```python
from build123d import *

# Parameters (mm, degrees)
SKETCH1_W           = 400
SKETCH1_H           = 1000
SKETCH1_W_2         = 360
SKETCH1_H_2         = 960
SKETCH1_H_3         = 20
BOSS_EXTRUDE1_DEPTH = 400
SKETCH2_W           = 400
SKETCH2_H           = 1000
BOSS_EXTRUDE2_DEPTH = 10


with BuildPart() as part:
    # Sketch1 → Boss-Extrude1 (new body)
    # profile 1 of 4: a face of its own
    with BuildSketch(Plane.XY):
        with Locations((0, 500)):
            Rectangle(SKETCH1_W, SKETCH1_H)
        with Locations((0, 500)):
            Rectangle(SKETCH1_W_2, SKETCH1_H_2, mode=Mode.SUBTRACT)
    # profile 2 of 4: a face of its own
    with BuildSketch(Plane.XY):
        with Locations((0, 740)):
            Rectangle(SKETCH1_W_2, SKETCH1_H_3)
    # profile 3 of 4: a face of its own
    with BuildSketch(Plane.XY):
        with Locations((0, 500)):
            Rectangle(SKETCH1_W_2, SKETCH1_H_3)
    # profile 4 of 4: a face of its own
    with BuildSketch(Plane.XY):
        with Locations((0, 260)):
            Rectangle(SKETCH1_W_2, SKETCH1_H_3)
    extrude(amount=BOSS_EXTRUDE1_DEPTH)

    # Sketch2 → Boss-Extrude2 (add)
    with BuildSketch(Plane(origin=(0, 0, 0), x_dir=(-1, 0, 0), z_dir=(0, 0, -1))):
        with Locations((0, 500)):
            Rectangle(SKETCH2_W, SKETCH2_H)
    extrude(amount=-BOSS_EXTRUDE2_DEPTH)


solid = part.part
```
Source: CAD feature listing. Evaluate the final solid. Frame: model axes, mm. A direction names the side the tool comes from. Give positions to 0.01 mm unless a question says otherwise; leave off trailing zeros. Loops run counter-clockwise (first coordinate to the right, second up) from the corner with the lowest first, then second, coordinate; pieces in that order, holes last. Notation, with made-up numbers: M -17,-5 L 27,-5 A20 ccw 27,32 Z; hole C 34.25,-1 d9. An arc over 180 degrees is marked long. Put each result on its own line as item: value.
Q1. Mould query, pull axis Y, two halves, no side actions, for faces 1 (the flat face through (-16, 502, 400)), 2 (the flat face through (-3, 1000, 197)), 3 (the flat face through (-3, 0, 197)), 4 (the flat face through (3, 137, 10)). Classes: released by +Y, released by -Y, zero draft, split by the parting line, or undercut.
Response values:
face 1: zero draft
face 2: released by +Y
face 3: released by -Y
face 4: undercut
Q2. Section C-C (y = 87). Return the cut outline in (x, z), and give its area (3 significant figures).
Response values:
outline: M -200,0 L 200,0 L 200,400 L 180,400 L 180,10 L -180,10 L -180,400 L -200,400 Z
area: 19,600 mm²
Q3. Line query: probe 1 along Y at (x, z) = (-130, 213); probe 2 along X at (y, z) = (282, 215); probe 3 along Z at (x, y) = (-179, 670.5). Output: solid intervals per line, ascending. Write a range as [from, to].
Response values:
probe 1: y = [0, 20], [250, 270], [490, 510], [730, 750], [980, 1000]
probe 2: x = [-200, -180], [180, 200]
probe 3: z = [0, 10]
Q4. Section B-B (x = -113.5). Return the cut outline in (y, z), and give its area (3 significant figures).
Response values:
outline: M 0,0 L 1000,0 L 1000,400 L 980,400 L 980,10 L 750,10 L 750,400 L 730,400 L 730,10 L 510,10 L 510,400 L 490,400 L 490,10 L 270,10 L 270,400 L 250,400 L 250,10 L 20,10 L 20,400 L 0,400 Z
area: 49,000 mm²
Q5. Section A-A (z = 205.5). Return the cut outline in (x, y).
Response values:
outline: M -200,0 L 200,0 L 200,1000 L -200,1000 Z; hole M -180,20 L 180,20 L 180,250 L -180,250 Z; hole M -180,270 L 180,270 L 180,490 L -180,490 Z; hole M -180,510 L 180,510 L 180,730 L -180,730 Z; hole M -180,750 L 180,750 L 180,980 L -180,980 Z
Q6. Pin query (flat end, axial travel): P1, Ø4, axis at x = 31.5, y = 286.5, coming from the -Z side; P2, Ø5, axis at x = -34, y = 775.5, coming from the +Z side. Return the tip coordinate at first contact, or that it passes through.
Response values:
P1: stops at z = 0
P2: stops at z = 10
Q7. Reachability of faces 5 (the flat face through (200, 493, 197)), 6 (the flat face through (-3, 510, 202)) from +Z, -Z, +X, -X, +Y, -Y: full face, straight path, thin tool, end or side. Return the list, or none.
Response values:
face 5: +Z, -Z, +X, +Y, -Y
face 6: +Z
